Can you work these out from the model? Positions are in its coordinate system, mm. Face numbers are marked on the shaded views. Coordinates: 2 decimals unless noted, no trailing zeros. Write each loop counter-clockwise with the first axis right and the second up, starting at its lowest first coordinate (ties: lowest second). Pieces come first, ordered by that corner, then holes. Notation, with made-up numbers: (82, 3) -> (117, 3) arc R20 cw to (117, 34) -> close; hole circle Ø8 at (-35, 59.25). An arc over 180 degrees is marked (long way). Use one line per item in the form item = value.
```python
from build123d import *

# Parameters (mm, degrees)
SKETCH_1_W                   = 200
SKETCH_1_H                   = 300
EXTRUDE_1_DEPTH              = 25
SKETCH_2_W                   = 12
SKETCH_2_H                   = 10
CUT_EXTRUDE_1_DEPTH          = 540.096466321
CUT_EXTRUDE_2_DEPTH          = 426.23522902
CHAMFER_2_SIZE               = 0.5
CHAMFER_3_SIZE               = 1
SKETCH_4_R                   = 20
CUT_EXTRUDE_3_DEPTH          = 589.833592792
CUT_EXTRUDE_4_DEPTH          = 540.096466321
M8X1_25_1_D                  = 6.8
HOLE_WIZARD_M6_1_D           = 6.4
HOLE_WIZARD_M6_1_CBORE_D     = 11
HOLE_WIZARD_M6_1_CBORE_DEPTH = 6
SKETCH_12_W                  = 1
SKETCH_12_H                  = 12
CUT_EXTRUDE_5_DEPTH          = 589.833592792
M8X1_25_2_D                  = 6.8
M8X1_25_2_DEPTH              = 22.25
M8X1_25_2_TIP                = 2.042926105
M6X1_0_1_D                   = 5
M6X1_0_1_DEPTH               = 17
M6X1_0_1_TIP                 = 1.502151548
M6X1_0_2_D                   = 5
CUT_EXTRUDE_6_DEPTH          = 589.833592792


with BuildPart() as part:
    # 草图1 → 凸台-拉伸1 (new body)
    with BuildSketch(Plane.XY):
        with Locations((210, 350)):
            Rectangle(SKETCH_1_W, SKETCH_1_H)
    extrude(amount=EXTRUDE_1_DEPTH)

    # 草图2 → 切除-拉伸1 (cut, through all)
    with BuildSketch(Plane.ZY.offset(-110)):
        with Locations((19, 495)):
            Rectangle(SKETCH_2_W, SKETCH_2_H)
        with Locations((19, 205)):
            Rectangle(SKETCH_2_W, SKETCH_2_H)
    extrude(amount=-CUT_EXTRUDE_1_DEPTH, mode=Mode.SUBTRACT)

    # 草图3 → 切除-拉伸2 (cut, through all)
    with BuildSketch(Plane(origin=(0, 490, 0), x_dir=(1, 0, 0), z_dir=(0, 1, 0))):
        Polygon((205.5, -25), (214.5, -25), (214.5, -19), (219.5, -19), (219.5, -13), (200.5, -13), (200.5, -19), (205.5, -19), align=None)
    extrude(amount=-CUT_EXTRUDE_2_DEPTH, mode=Mode.SUBTRACT)

    # 倒角2
    chamfer_2_edges = [part.edges().sort_by_distance(p)[0] for p in [
        (110, 500, 6.5),
        (310, 500, 6.5),
        (210, 500, 13),
        (310, 200, 6.5),
        (110, 200, 6.5),
        (210, 200, 13),
        (210, 500, 0),
        (210, 200, 0),
    ]]
    chamfer(chamfer_2_edges, length=CHAMFER_2_SIZE)

    # 倒角3
    chamfer_3_edges = [part.edges().sort_by_distance(p)[0] for p in [
        (110, 350, 25),
        (262.25, 490, 25),
        (310, 350, 25),
        (262.25, 210, 25),
        (157.75, 210, 25),
        (157.75, 490, 25),
        (205.5, 350, 25),
        (214.5, 350, 25),
    ]]
    chamfer(chamfer_3_edges, length=CHAMFER_3_SIZE)

    # 草图4 → 切除-拉伸3 (cut, through all)
    with BuildSketch(Plane.XY.offset(25)):
        with Locations((210, 350)):
            Circle(SKETCH_4_R)
    extrude(amount=-CUT_EXTRUDE_3_DEPTH, mode=Mode.SUBTRACT)

    # 草图5 → 切除-拉伸4 (cut, through all)
    with BuildSketch(Plane.ZY.offset(-110)):
        Polygon((25, 421), (25, 430), (19, 430), (19, 435), (13, 435), (13, 416), (19, 416), (19, 421), align=None)
        Polygon((13, 265), (19, 265), (19, 270), (25, 270), (25, 279), (19, 279), (19, 284), (13, 284), align=None)
    extrude(amount=-CUT_EXTRUDE_4_DEPTH, mode=Mode.SUBTRACT)

    # M8x1.25 螺纹孔1 (through all)
    with Locations(Plane.XY.offset(25)):
        with Locations((161, 350), (210, 399), (259, 350), (210, 301)):
            Hole(M8X1_25_1_D / 2)

    # M6 凹头盖螺钉的柱形沉头孔1 (through all)
    with Locations(Plane(origin=(0, 0, 0), x_dir=(-1, 0, 0), z_dir=(0, 0, -1))):
        with Locations((-125, 394.25), (-140, 394.25), (-140, 306.25), (-125, 306.25)):
            CounterBoreHole(HOLE_WIZARD_M6_1_D / 2, HOLE_WIZARD_M6_1_CBORE_D / 2, HOLE_WIZARD_M6_1_CBORE_DEPTH)

    # 草图12 → 切除-拉伸5 (cut, through all)
    with BuildSketch(Plane.XY.offset(25)):
        with Locations((309.5, 431)):
            Rectangle(SKETCH_12_W, SKETCH_12_H)
        with Locations((309.5, 269)):
            Rectangle(SKETCH_12_W, SKETCH_12_H)
    extrude(amount=-CUT_EXTRUDE_5_DEPTH, mode=Mode.SUBTRACT)

    # M8x1.25 螺纹孔2
    with Locations(Plane(origin=(309, 0, 0), x_dir=(0, 0, -1), z_dir=(1, 0, 0))):
        with Locations((-7, 431), (-7, 269)):
            Hole(M8X1_25_2_D / 2, depth=M8X1_25_2_DEPTH)
            with Locations((0, 0, -(M8X1_25_2_DEPTH + M8X1_25_2_TIP / 2))):  # 118° drill point
                Cone(0, M8X1_25_2_D / 2, M8X1_25_2_TIP, mode=Mode.SUBTRACT)

    # M6x1.0 螺纹孔1
    with Locations(Plane.ZY.offset(-110)):
        with Locations((7, 380), (7, 320)):
            Hole(M6X1_0_1_D / 2, depth=M6X1_0_1_DEPTH)
            with Locations((0, 0, -(M6X1_0_1_DEPTH + M6X1_0_1_TIP / 2))):  # 118° drill point
                Cone(0, M6X1_0_1_D / 2, M6X1_0_1_TIP, mode=Mode.SUBTRACT)

    # M6x1.0 螺纹孔2 (through all)
    with Locations(Plane.XY.offset(25)):
        with Locations((250, 467), (268, 449), (250, 233), (268, 251)):
            Hole(M6X1_0_2_D / 2)

    # 草图19 → 切除-拉伸6 (cut, through all)
    with BuildSketch(Plane.XY.offset(25)):
        Polygon((110, 358), (118, 358), (118, 363), (126, 363), (126, 337), (118, 337), (118, 342), (110, 342), align=None)
    extrude(amount=-CUT_EXTRUDE_6_DEPTH, mode=Mode.SUBTRACT)


solid = part.part
```
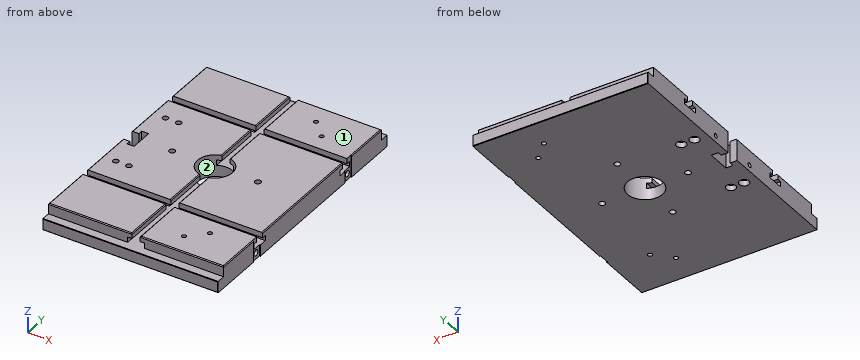
Q1. Thinking about a two-plate mould opening in X: for the marked faces 1 and 2, which applies, released by +X, released by -X, zero draft, split by the parting line, or undercut?
Return value:
face_1 = zero draft
face_2 = undercut
Q2. If I drill on line 1 (Y direction, x = 300.75, z = 7); line 2 (Y direction, x = 161, z = 18.5); line 3 (Y direction, x = 268, z = 19.75), over which ranges is the centre line in solid material (lowest first)? Write a range as from..to.
Return value:
line_1 = 200..265.6, 272.4..427.6, 434.4..500
line_2 = 210..265, 284..346.6, 353.4..416, 435..490
line_3 = 210..248.5, 253.5..270, 279..421, 430..446.5, 451.5..490
Q3. Will these pins go through, and if not, where does the flat tip stop? pin 1 (9 mm diameter, centred on x = 148.5, z = 18, fed in from -Y); pin 2 (1 mm diameter, centred on x = 177.5, y = 311.5, fed in from -Z); pin 3 (8.5 mm diameter, centred on x = 140, y = 306.25, fed in from -Z); pin 4 (6 mm diameter, centred on y = 433, z = 19.5, fed in from +X).
Return value:
pin_1 = 210
pin_2 = 0
pin_3 = 6
pin_4 = 309
Q4. Suppose I cut it at D-D (x = 140). Give the number of separate pieces and of enclosed holes in the cut face, then the cut area to 3 significant figures.
Return value:
separate_pieces = 3
enclosed_holes = 0
area = 6,550 mm2
Q5. Suppose I cut it at A-A (x = 210). Write out the boundary of the cut face in (y, z), then the cut area to 3 significant figures.
Return value:
outline = (200, 0.5) -> (200.5, 0) -> (297.6, 0) -> (297.6, 13) -> (200.5, 13) -> (200, 12.5) -> close; (304.4, 0) -> (330, 0) -> (330, 13) -> (304.4, 13) -> close; (370, 0) -> (395.6, 0) -> (395.6, 13) -> (370, 13) -> close; (402.4, 0) -> (499.5, 0) -> (500, 0.5) -> (500, 12.5) -> (499.5, 13) -> (402.4, 13) -> close
area = 3,200 mm2
Q6. Suppose I cut it at C-C (y = 459.5). Write out the boundary of the cut face in (x, z), then the cut area to 3 significant figures.
Return value:
outline = (110, 0) -> (310, 0) -> (310, 24) -> (309, 25) -> (215.5, 25) -> (214.5, 24) -> (214.5, 19) -> (219.5, 19) -> (219.5, 13) -> (200.5, 13) -> (200.5, 19) -> (205.5, 19) -> (205.5, 24) -> (204.5, 25) -> (111, 25) -> (110, 24) -> close
area = 4,830 mm2
